Build history of the part. All positions in model axes, mm. A direction names the side the tool comes from. Give positions to 0.01 mm unless a question says otherwise; leave off trailing zeros. Loops run counter-clockwise (first coordinate to the right, second up) from the corner with the lowest first, then second, coordinate; pieces in that order, holes last. Notation, with made-up numbers: (38, 20) -> (71, 20) arc R26 ccw to (71, 55) -> close; hole circle Ø10 at (40.25, 25.5). An arc over 180 degrees is marked (long way). Answer as a JSON object with one key per item and string values. Group by question number.
Q1. Band-saw the part on D-D, the plane x = -51. Write the cut outline in (y, z).
Q2. Drop flat-ended pins along their axis: pin 1 (4 mm diameter, centred on x = -42.88, y = -12.7, fed in from +Z); pin 2 (6 mm diameter, centred on x = 42.88, y = -12.7, fed in from -Z). Give the stop position or say it passes through.
Q3. Band-saw the part on A-A, the plane z = 9.25. Write the cut outline in (x, y).
Q4. Band-saw the part on C-C, the plane y = 0. Write the cut outline in (x, z).
Q5. Two-plate mould, pull along X, no slides. Class faces 1 (the flat face through (-9, -22.578, 13)), 2 (the flat face through (-108.382, 4, 23)), 3 (the cylindrical face through (40.849, -14.253, 1.431)), 4 (the cylindrical face through (40.849, -14.253, 24.009)): pulls with the +X half, pulls with the -X half, needs draft (parallel to the pull), parting line crosses it, or undercut.
Q6. Wall check: probe 1 along Y at (x, z) = (75.5, 9); probe 2 along Z at (x, y) = (50.5, -22); probe 3 along X at (y, z) = (0, 23.4). Give the ranges that are in metal, low to high. Write a range as from..to.
Q7. Band-saw the part on B-B, the plane x = 0. Write the cut outline in (y, z).
Q8. Tool access for faces 5 (the cylindrical face through (42.32, 10.21, 1.43)), 6 (the flat face through (-9, 15, 2.822)): list every direction of +Z, -Z, +X, -X, +Y, -Y with a clear straight run to the whole face (end or side of a thin tool).
Autodesk Inventor part; units mm, degrees
ref_plane "YZ Plane" through (0, 0, 0) normal (1, 0, 0) x (0, 1, 0)
ref_plane "XZ Plane" through (0, 0, 0) normal (0, 1, 0) x (-1, 0, 0)
ref_plane "XY Plane" through (0, 0, 0) normal (0, 0, 1) x (1, 0, 0)
sketch "Sketch1" plane through (0, 0, 0) normal (0, 0, 1) x (1, 0, 0)
  circle A0 centre (0, 0) radius 14.2875
  line L0 (88.4644, 25.4) -> (-108.3818, 25.4)
  line L1 (-108.3818, 25.4) -> (-108.3818, -25.4)
  line L2 (-108.3818, -25.4) -> (88.4644, -25.4)
  line L3 (88.4644, -25.4) -> (88.4644, 25.4)
  dimension "d0" = 28.575
  dimension "d4" = 50.8
  dimension "d15" = 88.4644
  dimension "d16" = 108.3818
extrude "Extrusion1" add sketch "Sketch1" along normal blind 25.4
sketch "Sketch2" plane through (88.4644, -25.4, 0) normal (1, 0, 0) x (0, 0, -1)
  line L0 (0, 50.8) -> (-25.4, 50.8)
  line L1 (0, 0) -> (-25.4, 0)
  line L2 (0, 50.8) -> (-25.4, 50.8)
  line L3 (-25.4, 50.8) -> (-25.4, 0)
  line L4 (-25.4, 0) -> (0, 0)
  line L5 (0, 0) -> (0, 50.8)
  line L6 (-22.5778, 2.8222) -> (-22.5778, 47.9778)
  line L7 (-22.5778, 47.9778) -> (-2.8222, 47.9778)
  line L8 (-2.8222, 47.9778) -> (-2.8222, 2.8222)
  line L9 (-2.8222, 2.8222) -> (-22.5778, 2.8222)
  point P0 (0, 25.4)
  dimension "d7" = 2.8222
extrude "Extrusion2" cut sketch "Sketch2" against normal blind 203.2 contours L6 L7 L8 L9
sketch "Sketch3" plane through (0, 0, 25.4) normal (0, 0, 1) x (1, 0, 0)
  circle A0 centre (42.8752, 12.7) radius 2.5527
  circle A1 centre (42.8752, -12.7) radius 2.5527
  circle A2 centre (-42.8752, 12.7) radius 2.5527
  circle A3 centre (-42.8752, -12.7) radius 2.5527
  point P0 (0, 0)
  dimension "d12" = 5.1054
extrude "Extrusion3" cut sketch "Sketch3" against normal blind 25.4
sketch "Sketch4" plane through (0, 0, 25.4) normal (0, 0, 1) x (1, 0, 0)
  point P0 (0, 0)
properties part number "gearboxsupportbar" material "Aluminum 6061"
Worked answers:
{
 "1": {"outline": "(-25.4, 0) -> (25.4, 0) -> (25.4, 25.4) -> (-25.4, 25.4) -> close; hole (-22.58, 2.82) -> (22.58, 2.82) -> (22.58, 22.58) -> (-22.58, 22.58) -> close"},
 "2": {"pin 1": "through", "pin 2": "z = 0"},
 "3": {"outline": "(-108.38, -25.4) -> (88.46, -25.4) -> (88.46, -22.58) -> (-108.38, -22.58) -> close; (-108.38, 22.58) -> (88.46, 22.58) -> (88.46, 25.4) -> (-108.38, 25.4) -> close"},
 "4": {"outline": "(-108.38, 0) -> (-14.29, 0) -> (-14.29, 2.82) -> (-108.38, 2.82) -> close; (-108.38, 22.58) -> (-14.29, 22.58) -> (-14.29, 25.4) -> (-108.38, 25.4) -> close; (14.29, 0) -> (88.46, 0) -> (88.46, 2.82) -> (14.29, 2.82) -> close; (14.29, 22.58) -> (88.46, 22.58) -> (88.46, 25.4) -> (14.29, 25.4) -> close"},
 "5": {"face 1": "needs draft", "face 2": "pulls with the -X half", "face 3": "undercut", "face 4": "undercut"},
 "6": {"probe 1": "-25.4..-22.58, 22.58..25.4", "probe 2": "0..2.82, 22.58..25.4", "probe 3": "-108.38..-14.29, 14.29..88.46"},
 "7": {"outline": "(-25.4, 0) -> (-14.29, 0) -> (-14.29, 2.82) -> (-22.58, 2.82) -> (-22.58, 22.58) -> (-14.29, 22.58) -> (-14.29, 25.4) -> (-25.4, 25.4) -> close; (14.29, 0) -> (25.4, 0) -> (25.4, 25.4) -> (14.29, 25.4) -> (14.29, 22.58) -> (22.58, 22.58) -> (22.58, 2.82) -> (14.29, 2.82) -> close"},
 "8": {"face 5": "+Z, -Z", "face 6": "+X, -X"}
}
